For this review, take the finished solid that the model builds, in its own axes (mm). A direction names the side the tool comes from. Coordinates: 2 decimals unless noted, no trailing zeros. Write each loop counter-clockwise with the first axis right and the second up, starting at its lowest first coordinate (ties: lowest second). Pieces come first, ordered by that corner, then holes.
```python
from build123d import *

# Parameters (mm, degrees)
PAD_DEPTH    = 20
POCKET_DEPTH = 18


with BuildPart() as part:
    # Sketch → Pad (new body)
    with BuildSketch(Plane.XY):
        Polygon((0, 0), (0, 90), (20, 90), (20, 40.00002), (40, 20), (90, 20), (90, 0), align=None)
    extrude(amount=PAD_DEPTH)

    # Sketch001 → Pocket (cut)
    with BuildSketch(Plane.XY.offset(20)):
        Polygon((3, 7), (3, 86), (18, 86), (18, 22.000015), align=None)
        Polygon((21.999985, 18), (86, 18), (86, 3), (7, 3), align=None)
    extrude(amount=-POCKET_DEPTH, mode=Mode.SUBTRACT)


solid = part.part
```
1) Consider section A-A (z = 13.75). Give the boundary of the cut face in (x, y).
2) For L1, parallel to X at y = 67, z = 12; L2, parallel to X at y = 12, z = 15.25, list the stretches that pass through material, from the lowest coordinate up.
3) Tool access review of faces 1 (the face through (20, 65, 10)), 2 (the face through (11, 15, 11)), 3 (the face through (10, 90, 10)): name each direction out of +Z, -Z, +X, -X, +Y, -Y from which nothing blocks a thin tool from reaching the whole face with its end or side.
4) Consider section D-D (x = 10.5). Give the boundary of the cut face in (y, z).
5) Clearance check with flat-ended pins moving along their axes: P1, Ø7.5, axis at x = 12, z = 11, coming from the -Y side; P2, Ø7.5, axis at x = 45.5, y = 9.5, coming from the +Z side; P3, Ø10, axis at x = 62, z = 9.5, coming from the +Y side; P4, Ø3, axis at x = 23, z = 8.5, coming from the +Y side. State where each tip first meets the part, or that it passes through.
6) Consider section C-C (x = 34). Give the boundary of the cut face in (y, z), then the cut area to 3 significant figures.
7) Consider section B-B (y = 64). Give the boundary of the cut face in (x, z).
Results:
1. outline: (0, 0) - (90, 0) - (90, 20) - (40, 20) - (20, 40) - (20, 90) - (0, 90) - close; hole (3, 7) - (18, 22) - (18, 86) - (3, 86) - close; hole (7, 3) - (86, 3) - (86, 18) - (22, 18) - close
2. L1: x = 0 to 3, 18 to 20
2. L2: x = 0 to 3, 8 to 16, 86 to 90
3. face 1: +Z, -Z, +X, +Y
3. face 2: +Z
3. face 3: +Z, -Z, +X, -X, +Y
4. outline: (0, 0) - (90, 0) - (90, 20) - (86, 20) - (86, 2) - (14.5, 2) - (14.5, 20) - (6.5, 20) - (6.5, 2) - (3, 2) - (3, 20) - (0, 20) - close
5. P1: stops at y = 0
5. P2: stops at z = 2
5. P3: stops at y = 20
5. P4: stops at y = 38.5
6. outline: (0, 0) - (26, 0) - (26, 20) - (18, 20) - (18, 2) - (3, 2) - (3, 20) - (0, 20) - close
6. area: 250 mm2
7. outline: (0, 0) - (20, 0) - (20, 20) - (18, 20) - (18, 2) - (3, 2) - (3, 20) - (0, 20) - close
